Part model, mm, in its own coordinate system. A direction names the side the tool comes from. Coordinates: 2 decimals unless noted, no trailing zeros. Loops run counter-clockwise (first coordinate to the right, second up) from the corner with the lowest first, then second, coordinate; pieces in that order, holes last. Notation, with made-up numbers: (-14, 12) - (14, 12) arc R20 ccw to (14, 48) - close; hole circle Ø5 at (60.25, 28). An arc over 180 degrees is marked (long way). Use a Markdown table: item, result. Add a question column.
1) Drop flat-ended pins along their axis: P1, Ø5, axis at x = 149, z = -30.5, coming from the -Y side; P2, Ø4.5, axis at x = 12.7, z = -75.946, coming from the -Y side. Give the stop position or say it passes through.
2) Pull direction Z, two halves, no side cores. Call faces 1 (the face through (78.867, 3, -64)), 2 (the face through (182, 3, 0)), 3 (the face through (0, 3, -63)): +Z half, -Z half, draft (parallel to the pull), parting line (faces both ways), or undercut.
3) Probe probe 1 along X at (y, z) = (2.5, -114.3); probe 2 along Z at (x, y) = (326.39, 3); probe 3 along Z at (x, y) = (118.5, 1.5) (3 decimals). List the from-to ranges inside material, lowest first. Write a range as [from, to].
4) Band-saw the part on A-A (x = 95.5). Give the cut face in (y, z) (3 decimals).
5) Band-saw the part on B-B (y = 5.25). Give the number of separate pieces and of enclosed holes in the cut face, plus the area to 3 significant figures.
6) Tool access for faces 4 (the face through (104, 3, -79.375)), 5 (the face through (182, 0, -64)): list every direction of +Z, -Z, +X, -X, +Y, -Y with a clear straight run to the whole face (end or side of a thin tool).
from build123d import *

# Parameters (mm, degrees)
SKETCH1_W           = 368.3
SKETCH1_H           = 127
SKETCH1_R           = 2.5527
BOSS_EXTRUDE1_DEPTH = 6.35
CUT_EXTRUDE1_REACH  = 391.633
SKETCH2_R           = 2.5527
SKETCH2_W           = 50.8
SKETCH2_H           = 31.75


with BuildPart() as part:
    # Sketch1 → Boss-Extrude1 (new body)
    with BuildSketch(Plane(origin=(0, 0, 0), x_dir=(1, 0, 0), z_dir=(0, 1, 0))):
        with Locations((184.15, 63.5)):
            Rectangle(SKETCH1_W, SKETCH1_H)
        with Locations(Location((326.39, 12.7, 0), (0, 0, 270))):
            Circle(SKETCH1_R, mode=Mode.SUBTRACT)
        with Locations(Location((41.91, 12.7, 0), (0, 0, 270))):
            Circle(SKETCH1_R, mode=Mode.SUBTRACT)
        with Locations(Location((41.91, 114.3, 0), (0, 0, 270))):
            Circle(SKETCH1_R, mode=Mode.SUBTRACT)
        with Locations(Location((326.39, 114.3, 0), (0, 0, 270))):
            Circle(SKETCH1_R, mode=Mode.SUBTRACT)
        with Locations(Location((215.646, 12.7, 0), (0, 0, 270))):
            Circle(SKETCH1_R, mode=Mode.SUBTRACT)
        with Locations(Location((152.654, 12.7, 0), (0, 0, 270))):
            Circle(SKETCH1_R, mode=Mode.SUBTRACT)
        with Locations(Location((215.646, 114.3, 0), (0, 0, 270))):
            Circle(SKETCH1_R, mode=Mode.SUBTRACT)
        with Locations(Location((152.654, 114.3, 0), (0, 0, 270))):
            Circle(SKETCH1_R, mode=Mode.SUBTRACT)
        with Locations(Location((12.7, 75.946, 0), (0, 0, 270))):
            Circle(SKETCH1_R, mode=Mode.SUBTRACT)
        with Locations(Location((355.6, 51.054, 0), (0, 0, 270))):
            Circle(SKETCH1_R, mode=Mode.SUBTRACT)
    extrude(amount=BOSS_EXTRUDE1_DEPTH)

    # Sketch2 → Cut-Extrude1 (cut, up to next)
    with BuildSketch(Plane.XZ, mode=Mode.PRIVATE) as cut_extrude1_sk1:
        with Locations(Location((76.2, -44.958, 0), (0, 0, 270))):
            Circle(SKETCH2_R)
    cut_extrude1_tool1 = extrude(cut_extrude1_sk1.sketch, amount=-CUT_EXTRUDE1_REACH, mode=Mode.PRIVATE) & part.part
    # Sketch2 → Cut-Extrude1 (cut, up to next)
    with BuildSketch(Plane.XZ, mode=Mode.PRIVATE) as cut_extrude1_sk2:
        with Locations(Location((132.334, -82.042, 0), (0, 0, 270))):
            Circle(SKETCH2_R)
    cut_extrude1_tool2 = extrude(cut_extrude1_sk2.sketch, amount=-CUT_EXTRUDE1_REACH, mode=Mode.PRIVATE) & part.part
    # Sketch2 → Cut-Extrude1 (cut, up to next)
    with BuildSketch(Plane.XZ, mode=Mode.PRIVATE) as cut_extrude1_sk3:
        with Locations((104.267, -63.5)):
            Rectangle(SKETCH2_W, SKETCH2_H)
    cut_extrude1_tool3 = extrude(cut_extrude1_sk3.sketch, amount=-CUT_EXTRUDE1_REACH, mode=Mode.PRIVATE) & part.part
    add(cut_extrude1_tool1.solids().sort_by_distance((76.2, 0, -44.958))[0], mode=Mode.SUBTRACT)
    add(cut_extrude1_tool2.solids().sort_by_distance((132.334, 0, -82.042))[0], mode=Mode.SUBTRACT)
    add(cut_extrude1_tool3.solids().sort_by_distance((104.267, 0, -63.5))[0], mode=Mode.SUBTRACT)


solid = part.part
Answer block:
| question | item | result |
|---|---|---|
| 1 | P1 | y = 0 |
| 1 | P2 | through |
| 2 | face 1 | undercut |
| 2 | face 2 | +Z half |
| 2 | face 3 | draft |
| 3 | probe 1 | [0, 39.36], [44.46, 150.1], [155.21, 213.09], [218.2, 323.84], [328.94, 368.3] |
| 3 | probe 2 | [-127, -116.85], [-111.75, -15.25], [-10.15, 0] |
| 3 | probe 3 | [-127, -79.375], [-47.625, 0] |
| 4 | outline | (0, -127) - (6.35, -127) - (6.35, -79.375) - (0, -79.375) - close; (0, -47.625) - (6.35, -47.625) - (6.35, 0) - (0, 0) - close |
| 5 | separate pieces | 1 |
| 5 | enclosed holes | 13 |
| 5 | area | 44,900 mm2 |
| 6 | face 4 | +Y, -Y |
| 6 | face 5 | +Z, -Z, +X, -X, -Y |
